Can you work these out from the model? Positions are in its coordinate system, mm. A direction names the side the tool comes from. Coordinates: 2 decimals unless noted, no trailing zeros. Write each loop counter-clockwise with the first axis right and the second up, starting at its lowest first coordinate (ties: lowest second). Pieces come first, ordered by that corner, then holes. Notation, with made-up numbers: (76, 75.25) -> (129, 75.25) arc R21 cw to (129, 86.25) -> close; hole circle Ø4 at (6, 74). An arc over 180 degrees is marked (long way). Use one line per item in the form item = value.
```python
from build123d import *

# Parameters (mm, degrees)
SKETCH1_R           = 2
BOSS_EXTRUDE2_DEPTH = 1


with BuildPart() as part:
    # Sketch1 → Boss-Extrude2 (new body)
    with BuildSketch(Plane(origin=(0, 0, 0), x_dir=(1, 0, 0), z_dir=(0, 1, 0))):
        with BuildLine():
            Line((0, 40), (15, 40))
            Line((15, 40), (15, 0))
            Line((15, 0), (15, -15))
            Line((15, -15), (-52, -15))
            Line((-52, -15), (-52, 58))
            Line((-52, 58), (-37, 58))
            Line((-37, 58), (-35, 58))
            Line((-35, 58), (-35, 30))
            Line((-35, 30), (-37, 30))
            Line((-37, 30), (-37, 5))
            ThreePointArc((-37, 5), (-36.121320344, 2.878679656), (-34, 2))
            Line((-34, 2), (-6, 2))
            ThreePointArc((-6, 2), (-3.878679656, 2.878679656), (-3, 5))
            Line((-3, 5), (-3, 40))
            Line((-3, 40), (0, 40))
        make_face()
        with Locations((6, 32)):
            Circle(SKETCH1_R, mode=Mode.SUBTRACT)
        with Locations((6, 17)):
            Circle(SKETCH1_R, mode=Mode.SUBTRACT)
        with Locations((-43, 53)):
            Circle(SKETCH1_R, mode=Mode.SUBTRACT)
        with Locations((-43, 33)):
            Circle(SKETCH1_R, mode=Mode.SUBTRACT)
        with Locations((-37, -6)):
            Circle(SKETCH1_R, mode=Mode.SUBTRACT)
        with Locations((-2, -6)):
            Circle(SKETCH1_R, mode=Mode.SUBTRACT)
    extrude(amount=BOSS_EXTRUDE2_DEPTH)


solid = part.part
```
Q1. For faces 1 (the flat face through (-18, 1, 2)), 2 (the cylindrical face through (-3.9, 0.49, -2.86)), 3 (the cylindrical face through (-36.14, 0.49, -2.9)), which set-ups out of +Z, -Z, +X, -X, +Y, -Y let a thin tool reach every point of the face, with its end or its side?
Return value:
face_1 = +Z, -Z, +X, -X, +Y
face_2 = -Z, +Y, -Y
face_3 = +Y, -Y
Q2. If I drill on line 1 (X direction, y = 0.35, z = -17); line 2 (Z direction, x = -43, y = 0.7); line 3 (Z direction, x = 6, y = 0.6), over which ranges is the centre line in solid material (lowest first)? Write a range as from..to.
Return value:
line_1 = -52..-37, -3..4, 8..15
line_2 = -58..-55, -51..-35, -31..15
line_3 = -40..-34, -30..-19, -15..15
Q3. Suppose I cut it at A-A (x = 6). Write out the boundary of the cut face in (y, z).
Return value:
outline = (0, -40) -> (1, -40) -> (1, -34) -> (0, -34) -> close; (0, -30) -> (1, -30) -> (1, -19) -> (0, -19) -> close; (0, -15) -> (1, -15) -> (1, 15) -> (0, 15) -> close
Q4. Suppose I cut it at C-C (y = 0.5). Write out the boundary of the cut face in (x, z), then the cut area to 3 significant figures.
Return value:
outline = (-52, -58) -> (-35, -58) -> (-35, -30) -> (-37, -30) -> (-37, -5) arc R3 cw to (-34, -2) -> (-6, -2) arc R3 cw to (-3, -5) -> (-3, -40) -> (15, -40) -> (15, 15) -> (-52, 15) -> close; hole circle Ø4 at (-43, -53); hole circle Ø4 at (-43, -33); hole circle Ø4 at (-37, 6); hole circle Ø4 at (-2, 6); hole circle Ø4 at (6, -32); hole circle Ø4 at (6, -17)
area = 2,650 mm2
Q5. Suppose I cut it at D-D (x = -38). Write out the boundary of the cut face in (y, z).
Return value:
outline = (0, -58) -> (1, -58) -> (1, 4.27) -> (0, 4.27) -> close; (0, 7.73) -> (1, 7.73) -> (1, 15) -> (0, 15) -> close
Q6. Thinking about a two-plate mould opening in X: for faces 4 (the cylindrical face through (5.74, 0.493, -18.983)), 5 (the flat face through (-18, 0, 2)), which applies, released by +X, released by -X, zero draft, split by the parting line, or undercut?
Return value:
face_4 = undercut
face_5 = zero draft
Q7. Will these pins go through, and if not, where does the flat tip stop? pin 1 (10 mm diameter, centred on x = -11, z = -21, fed in from +Y); pin 2 (0.5 mm diameter, centred on x = -19.5, y = 0.5, fed in from -Z).
Return value:
pin_1 = through
pin_2 = -2
